Build history of the part. All positions in model axes, mm. A direction names the side the tool comes from. Coordinates: 2 decimals unless noted, no trailing zeros. Write each loop counter-clockwise with the first axis right and the second up, starting at its lowest first coordinate (ties: lowest second). Pieces come first, ordered by that corner, then holes.
```python
from build123d import *

# Parameters (mm, degrees)
SKETCH023_W             = 7.6
SKETCH023_H             = 7.6
PAD012_DEPTH            = 2
SKETCH024_R             = 1.6
PAD013_DEPTH            = 1.696
BODY042_PLACEMENT_ANGLE = 180
SKETCH020_W             = 30
SKETCH020_H             = 30
PAD010_DEPTH            = 4
CHAMFER_SIZE            = 3
FILLET011_R             = 2
SKETCH021_W             = 7.6
SKETCH021_H             = 7.6
PAD011_DEPTH            = 8.4
SKETCH022_R             = 2
POCKET004_DEPTH         = 6.7


with BuildPart() as obj1:
    # Sketch023 → Pad012 (new body)
    with BuildSketch(Plane.XY):
        with Locations((-11.2, -11.2)):
            Rectangle(SKETCH023_W, SKETCH023_H)
    extrude(amount=-PAD012_DEPTH)

    # Sketch024 (on Face6 of Pad012) → Pad013 (join)
    with BuildSketch(Plane(origin=(0, 0, -2), x_dir=(1, 0, 0), z_dir=(0, 0, -1))):
        with Locations((-11, 11)):
            Circle(SKETCH024_R)
    extrude(amount=PAD013_DEPTH)


with BuildPart() as obj1_1:
    # Body029 placement: moved
    add(obj1.part.moved(Location((0, 0, -12.4))))


with BuildPart() as obj2:
    # Body043 base: copy of obj1
    add(obj1_1.part)


with BuildPart() as body044:
    # Body042 base: copy of obj1
    add(obj1_1.part)


with BuildPart() as body044_1:
    # Body042 placement: moved
    add(body044.part.rotate(Axis((0, 0, 0), (0, 0, 1)), BODY042_PLACEMENT_ANGLE))


with BuildPart() as fusion_sockettop:
    # Sketch020 → Pad010 (new body)
    with BuildSketch(Plane.XY):
        Rectangle(SKETCH020_W, SKETCH020_H)
        Polygon((0, 8), (-5.656854, 5.656854), (-8, 0), (-5.656854, -5.656854), (0, -8), (5.656854, -5.656854), (8, 0), (5.656854, 5.656854), align=None, mode=Mode.SUBTRACT)
    extrude(amount=-PAD010_DEPTH)

    # Chamfer
    chamfer_edges = [fusion_sockettop.edges().sort_by_distance(p)[0] for p in [
        (2.828427, 6.828427, 0),
        (6.828427, 2.828427, 0),
        (6.828427, -2.828427, 0),
        (2.828427, -6.828427, 0),
        (-2.828427, -6.828427, 0),
        (-6.828427, -2.828427, 0),
        (-6.828427, 2.828427, 0),
        (-2.828427, 6.828427, 0),
    ]]
    chamfer(chamfer_edges, length=CHAMFER_SIZE)

    # Fillet011
    fillet011_edges = [fusion_sockettop.edges().sort_by_distance(p)[0] for p in [
        (-6.804905, 6.804905, -1.5),
        (0, 9.623588, -1.5),
        (6.804905, 6.804905, -1.5),
        (9.623588, 0, -1.5),
        (-6.804905, -6.804905, -1.5),
        (-9.623588, 0, -1.5),
        (0, -9.623588, -1.5),
        (6.804905, -6.804905, -1.5),
    ]]
    fillet(fillet011_edges, radius=FILLET011_R)

    # Sketch021 (on Face4 of Fillet011) → Pad011 (join)
    with BuildSketch(Plane(origin=(0, 0, -4), x_dir=(1, 0, 0), z_dir=(0, 0, -1))):
        with Locations((-11.2, -11.2)):
            Rectangle(SKETCH021_W, SKETCH021_H)
        with Locations((11.2, -11.2)):
            Rectangle(SKETCH021_W, SKETCH021_H)
        with Locations((11.2, 11.2)):
            Rectangle(SKETCH021_W, SKETCH021_H)
        with Locations((-11.2, 11.2)):
            Rectangle(SKETCH021_W, SKETCH021_H)
    extrude(amount=PAD011_DEPTH)

    # Sketch022 (on Face43 of Pad011) → Pocket004 (cut)
    with BuildSketch(Plane(origin=(0, 0, -12.4), x_dir=(1, 0, 0), z_dir=(0, 0, -1))):
        with Locations((-11, 11)):
            Circle(SKETCH022_R)
        with Locations((11, 11)):
            Circle(SKETCH022_R)
        with Locations((11, -11)):
            Circle(SKETCH022_R)
        with Locations((-11, -11)):
            Circle(SKETCH022_R)
    extrude(amount=-POCKET004_DEPTH, mode=Mode.SUBTRACT)

    # Boolean003: union obj2, Body044
    add(obj2.part)
    add(body044_1.part)


solid = fusion_sockettop.part
```
1. Flat gauge pins, fed straight in: pin 1 (6 mm diameter, centred on y = 1.5, z = -4.5, fed in from +X); pin 2 (8.5 mm diameter, centred on x = -12.5, y = 10, fed in from -Z); pin 3 (2 mm diameter, centred on x = 11, y = -10.5, fed in from -Z); pin 4 (8 mm diameter, centred on x = 2.5, y = 5, fed in from +Z). Where does each tip first touch, or does it go through?
Computed values:
pin 1: stops at x = 15
pin 2: stops at z = -12.4
pin 3: stops at z = -5.7
pin 4: stops at z = -0.81
2. 3-axis set-ups, long thin cutter, end or side, ignore diameter. For faces 1 (the face through (-8.21, 3.46, -1.48)), 2 (the face through (11, -7.4, -8)), 3 (the face through (-7.4, 11, -8)), 4 (the face through (2.789, -6.845, -3.562)): which of +Z, -Z, +X, -X, +Y, -Y reach the whole face in a straight line?
Computed values:
face 1: +Z
face 2: -Z, +X, -X
face 3: -Z, +Y, -Y
face 4: +Z, -Z
3. Saw through at D-D on y = -11.75. List the corners of the cut face in (x, z), plus the area to 3 significant figures.
Computed values:
outline: (-15, -14.4) - (-12.41, -14.4) - (-12.41, -16.1) - (-9.59, -16.1) - (-9.59, -14.4) - (-7.4, -14.4) - (-7.4, -4) - (7.4, -4) - (7.4, -12.4) - (9.15, -12.4) - (9.15, -5.7) - (12.85, -5.7) - (12.85, -12.4) - (15, -12.4) - (15, 0) - (-15, 0) - close; hole (-12.85, -12.4) - (-9.15, -12.4) - (-9.15, -5.7) - (-12.85, -5.7) - close
area: 218 mm2
4. Probe line 1 along X through (y, z) = (11, -10.5); line 2 along Y through (x, z) = (-2.5, -0.75). List the from-to ranges inside material, lowest first.
Computed values:
line 1: x = -15 to -13, -9 to -7.4, 7.4 to 9, 13 to 15
line 2: y = -15 to -9.4, 9.4 to 15
5. Saw through at B-B on x = -3.5. List the corners of the cut face in (y, z).
Computed values:
outline: (-15, -4) - (-6.55, -4) - (-6.55, -3) - (-9.8, 0) - (-15, 0) - close; (6.55, -4) - (15, -4) - (15, 0) - (9.8, 0) - (6.55, -3) - close
6. Saw through at A-A on z = -9.25. List the corners of the cut face in (x, y), plus the area to 3 significant figures.
Computed values:
outline: (-15, -15) - (-7.4, -15) - (-7.4, -7.4) - (-15, -7.4) - close; (-15, 7.4) - (-7.4, 7.4) - (-7.4, 15) - (-15, 15) - close; (7.4, -15) - (15, -15) - (15, -7.4) - (7.4, -7.4) - close; (7.4, 7.4) - (15, 7.4) - (15, 15) - (7.4, 15) - close; hole circle Ø4 at (-11, -11); hole circle Ø4 at (-11, 11); hole circle Ø4 at (11, -11); hole circle Ø4 at (11, 11)
area: 181 mm2
7. Saw through at C-C on y = 4. List the corners of the cut face in (x, z).
Computed values:
outline: (-15, -4) - (-6.34, -4) - (-6.34, -3) - (-9.59, 0) - (-15, 0) - close; (6.34, -4) - (15, -4) - (15, 0) - (9.59, 0) - (6.34, -3) - close
8. Mould opens along X. For faces 5 (the face through (0, 15, -2)), 6 (the face through (-6.845, -2.789, -3.562)), 7 (the face through (-11, 11, -5.7)) say: +X half, -X half, draft (parallel to the pull), parting line (faces both ways), or undercut.
Computed values:
face 5: draft
face 6: undercut
face 7: undercut
